from build123d import *

# Parameters (mm, degrees)
SKETCH1_R               = 7.5
BOSS_EXTRUDE1_DEPTH     = 82.685
CUT_EXTRUDE2_DEPTH      = 84.362516907
CUT_EXTRUDE3_DEPTH      = 84.362517024
CUT_EXTRUDE4_DEPTH      = 84.624513422
CUT_EXTRUDE4_DEPTH_BACK = 84.624513422
SKETCH8_R               = 2.5
FILLET1_R               = 1
FILLET1_OF_MIRROR2_R    = 1
SKETCH9_R               = 3
CUT_EXTRUDE5_DEPTH      = 10


with BuildPart() as part:
    # Sketch1 → Boss-Extrude1 (new, symmetric)
    with BuildSketch(Plane.XY):
        Circle(SKETCH1_R)
    extrude(amount=BOSS_EXTRUDE1_DEPTH, both=True)

    # Sketch6 → Cut-Extrude2 (cut, symmetric)
    with BuildSketch(Plane(origin=(0, 0, 0), x_dir=(0, 0, -1), z_dir=(1, 0, 0))):
        with BuildLine():
            Line((82.685, 0), (82.685, 7.5))
            Line((82.685, 7.5), (76.685, 7.5))
            ThreePointArc((76.685, 7.5), (81.000428973, 4.802343178), (82.685, 0))
        make_face()
        with BuildLine():
            Line((82.685, -7.5), (82.685, 0))
            ThreePointArc((82.685, 0), (81.000428973, -4.802343178), (76.685, -7.5))
            Line((76.685, -7.5), (82.685, -7.5))
        make_face()
    cut_extrude2 = extrude(amount=CUT_EXTRUDE2_DEPTH, both=True, mode=Mode.SUBTRACT)

    # Sketch7 → Cut-Extrude3 (cut, symmetric)
    with BuildSketch(Plane(origin=(0, 0, 0), x_dir=(1, 0, 0), z_dir=(0, 1, 0))):
        Polygon((-2.5, 82.685), (-2.5, 65.685), (-7.5, 64.803365096), (-7.5, 82.685), align=None)
        Polygon((7.5, 82.685), (2.5, 82.685), (2.5, 65.685), (7.5, 64.803365096), align=None)
    cut_extrude3 = extrude(amount=CUT_EXTRUDE3_DEPTH, both=True, mode=Mode.SUBTRACT)

    # Sketch8 → Cut-Extrude4 (cut, two sides: drawn at the far end of the back side and taken through both)
    with BuildSketch(Plane(origin=(-2.5, 0, 0), x_dir=(0, 0, -1), z_dir=(1, 0, 0)).offset(-CUT_EXTRUDE4_DEPTH_BACK)):
        with Locations((74.9975, 0)):
            Circle(SKETCH8_R)
    extrude(amount=CUT_EXTRUDE4_DEPTH + CUT_EXTRUDE4_DEPTH_BACK, mode=Mode.SUBTRACT)

    # Fillet1
    fillet1_edges = [part.edges().sort_by_distance(p)[0] for p in [
        (-2.5, 0, -65.685),
        (2.5, 0, -65.685),
    ]]
    fillet(fillet1_edges, radius=FILLET1_R)

    # Mirror2: Cut-Extrude2, Cut-Extrude3 across plane
    add(cut_extrude2.mirror(Plane.XY), mode=Mode.SUBTRACT)
    add(cut_extrude3.mirror(Plane.XY), mode=Mode.SUBTRACT)

    # Fillet1 of Mirror2
    fillet1_of_mirror2_edges = [part.edges().sort_by_distance(p)[0] for p in [
        (-2.5, 0, 65.685),
        (2.5, 0, 65.685),
    ]]
    fillet(fillet1_of_mirror2_edges, radius=FILLET1_OF_MIRROR2_R)

    # Sketch9 → Cut-Extrude5 (cut)
    with BuildSketch(Plane(origin=(2.5, 0, 0), x_dir=(0, 0, -1), z_dir=(1, 0, 0))):
        with Locations((-74.9975, 0)):
            Circle(SKETCH9_R)
    extrude(amount=-CUT_EXTRUDE5_DEPTH, mode=Mode.SUBTRACT)


solid = part.part
Verification items for the finished model (mm, model axes). A direction names the side the tool comes from. Round coordinates to 2 decimals unless told otherwise and drop trailing zeros. Order: outer loops, then holes, each group sorted by start corner. A loop starts at its lowest first (then second) coordinate and runs counter-clockwise, first axis right, second up. Notation, with made-up numbers: (85.5, -37) -> (110.5, -37) arc R16 ccw to (110.5, -27) -> close; hole circle Ø11 at (86.25, 14). An arc over 180 degrees is marked (long way). Put each result on its own line as item: value.
1) Section check A-A (x = 0). Record the cut outline in (y, z) (1 decimal), then the cut area to 3 significant figures.
Final values:
outline: (-7.5, -76.7) arc R7.7 ccw to (7.5, -76.7) -> (7.5, 76.7) arc R7.7 ccw to (-7.5, 76.7) -> close; hole circle Ø6 at (0, 75); hole circle Ø5 at (0, -75)
area: 2,390 mm^2
2) Depth check by flat-ended pin: pin 1 (6.5 mm diameter, centred on y = 0, z = -75, fed in from -X); pin 2 (1.5 mm diameter, centred on x = -1, z = 2.5, fed in from +Y); pin 3 (7 mm diameter, centred on y = -1.5, z = 73.5, fed in from +X). Enter the tip coordinate at first touch or a pass-through.
Final values:
pin 1: stops at x = -2.5
pin 2: stops at y = 7.5
pin 3: stops at x = 2.5
3) Mould release check, pull along Z, two halves, no side actions. Record for faces 1 (the cylindrical face through (-0.035, 0.751, -77.382)), 2 (the flat face through (-4.92, -0.09, 65.26)), 3 (the flat face through (2.5, 2, -73)): +Z half, -Z half, draft (parallel to the pull), parting line (faces both ways), or undercut.
Final values:
face 1: undercut
face 2: +Z half
face 3: draft
4) Set-up check for faces 4 (the flat face through (-2.5, -2, -73)), 5 (the flat face through (-2.5, 0, 71)), 6 (the flat face through (4.92, 0.09, -65.26)), 7 (the flat face through (2.5, 0, 71)): record each of +Z, -Z, +X, -X, +Y, -Y from which the full face is reachable in a straight line by a thin tool's end or side.
Final values:
face 4: -Z, -X, +Y, -Y
face 5: +Z, -X, +Y, -Y
face 6: -Z, +X, +Y, -Y
face 7: +Z, +X, +Y, -Y
5) Section check B-B (y = 4.75). Record the cut outline in (x, z), then the cut area to 3 significant figures.
Final values:
outline: (-5.8, -65.1) -> (-3.33, -65.54) arc R1 cw to (-2.5, -66.52) -> (-2.5, -81.04) -> (2.5, -81.04) -> (2.5, -66.52) arc R1 cw to (3.33, -65.54) -> (5.8, -65.1) -> (5.8, 65.1) -> (3.33, 65.54) arc R1 cw to (2.5, 66.52) -> (2.5, 81.04) -> (-2.5, 81.04) -> (-2.5, 66.52) arc R1 cw to (-3.33, 65.54) -> (-5.8, 65.1) -> close
area: 1,680 mm^2
6) Section check C-C (z = 33). Record the cut outline in (x, y), then the cut area to 3 significant figures.
Final values:
outline: circle Ø15 at (0, 0)
area: 177 mm^2
7) Material ranges on line 1 (Z direction, x = 1, y = 0.25); line 2 (X direction, y = 2.75, z = 71.5); line 3 (Y direction, x = 0.25, z = 37), recorded low to high.
Final values:
line 1: z = -82.68 to -77.48, -72.51 to 72.01, 77.99 to 82.68
line 2: x = -2.5 to 2.5
line 3: y = -7.5 to 7.5
